Part print with two shaded views. Sizes in mm from the minimum x, y, z corner. Coordinates: 2 decimals unless noted, no trailing zeros. Write each loop counter-clockwise with the first axis right and the second up, starting at its lowest first coordinate (ties: lowest second). Pieces come first, ordered by that corner, then holes. Notation, with made-up numbers: (50.25, 89) - (92.25, 89) arc R20 cw to (92.25, 101) - close; hole circle Ø4 at (-16, 22.25). An arc over 180 degrees is marked (long way). Answer in a Markdown table with one row per item. Add a question column.
Q1. Band-saw the part on B-B (x = 43.5). List the corners of the cut face in (y, z).
Q2. Band-saw the part on A-A (y = 38.1). List the corners of the cut face in (x, z), and give its area (3 significant figures).
Q3. Band-saw the part on C-C (z = 68.5). List the corners of the cut face in (x, y), and give its area (3 significant figures).
Q4. Pin check, flat tip, straight feed: pin 1 (2 mm diameter, centred on x = 53, z = 76, fed in from -Y). Stop position of the tip, or through.
Q5. Band-saw the part on D-D (y = 76). List the corners of the cut face in (x, z), and give its area (3 significant figures).
Q6. Drill centre lines: line 1 along X through (y, z) = (38.1, 7.5); line 2 along Y through (x, z) = (59.5, 8); line 3 along Y through (x, z) = (62, 60). Where is each one in solid material? Low to high. Write a range as from..to.
Q7. Two-plate mould, pull along Z, no slides. Class the marked faces 1, 2 and 3: +Z half, -Z half, draft (parallel to the pull), parting line (faces both ways), or undercut.
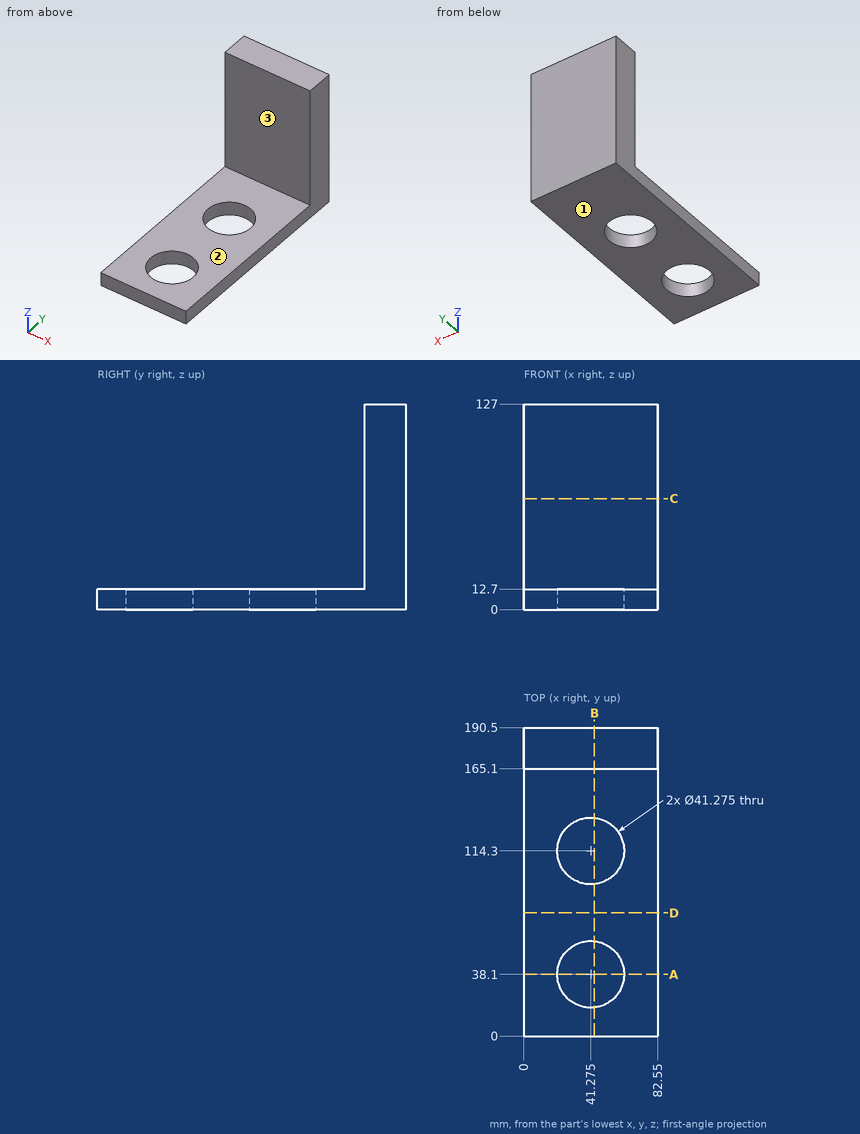
Checked values:
| question | item | result |
|---|---|---|
| 1 | outline | (0, 0) - (17.58, 0) - (17.58, 12.7) - (0, 12.7) - close; (58.62, 0) - (93.78, 0) - (93.78, 12.7) - (58.62, 12.7) - close; (134.82, 0) - (190.5, 0) - (190.5, 127) - (165.1, 127) - (165.1, 12.7) - (134.82, 12.7) - close |
| 2 | outline | (0, 0) - (20.64, 0) - (20.64, 12.7) - (0, 12.7) - close; (61.91, 0) - (82.55, 0) - (82.55, 12.7) - (61.91, 12.7) - close |
| 2 | area | 524 mm² |
| 3 | outline | (0, 165.1) - (82.55, 165.1) - (82.55, 190.5) - (0, 190.5) - close |
| 3 | area | 2,100 mm² |
| 4 | pin 1 | stops at y = 165.1 |
| 5 | outline | (0, 0) - (82.55, 0) - (82.55, 12.7) - (0, 12.7) - close |
| 5 | area | 1,050 mm² |
| 6 | line 1 | x = 0..20.64, 61.91..82.55 |
| 6 | line 2 | y = 0..28.42, 47.78..104.62, 123.98..190.5 |
| 6 | line 3 | y = 165.1..190.5 |
| 7 | face 1 | -Z half |
| 7 | face 2 | +Z half |
| 7 | face 3 | draft |
